Could you check a few things on this model? Use its own coordinates, in mm. A direction names the side the tool comes from. Coordinates: 2 decimals unless noted, no trailing zeros. Order: outer loops, then holes, each group sorted by start corner. A loop starts at its lowest first (then second) coordinate and runs counter-clockwise, first axis right, second up. Notation, with made-up numbers: (53.5, 41.25) - (84.5, 41.25) arc R28 ccw to (84.5, 59.25) - close; hole circle Ø4 at (83, 71). An arc over 180 degrees is marked (long way). One line per item, written item: value. Start each with the question number.
from build123d import *

# Parameters (mm, degrees)
BOSS_EXTRUDE1_DEPTH    = 25.4
CONVERT_SOLID1_DEPTH   = 25.4
CONVERT_SOLID1_2_DEPTH = 25.4
SKETCH7_R              = 2.5019
CUT_EXTRUDE1_DEPTH     = 39.1
FILLET1_R              = 2.54
SKETCH8_R              = 1.89865
CUT_EXTRUDE2_DEPTH     = 38.265357908


# Read off the part's stored shape, not the designer's step: Convert-Solid1
with BuildPart() as part:
    # Sketch2 → Boss-Extrude1 (new body)
    with BuildSketch(Plane.XY):
        Polygon((0, 0), (0, 25.4), (1.27, 25.4), (1.27, 1.27), (12.7, 1.27), (12.7, 0), align=None)
    extrude(amount=BOSS_EXTRUDE1_DEPTH)

    # Convert-Solid1 outline → Convert-Solid1 (cut)
    with BuildSketch(Plane.XY):
        with BuildLine():
            ThreePointArc((2.54, 0), (0.743948776, 0.743948776), (0, 2.54))
            Line((0, 2.54), (0, 0))
            Line((0, 0), (2.54, 0))
        make_face()
    extrude(amount=CONVERT_SOLID1_DEPTH, mode=Mode.SUBTRACT)

    # Convert-Solid1 2 outline → Convert-Solid1 2 (add)
    with BuildSketch(Plane.XY):
        with BuildLine():
            ThreePointArc((2.54, 1.27), (1.641974388, 1.641974388), (1.27, 2.54))
            Line((1.27, 2.54), (1.27, 1.27))
            Line((1.27, 1.27), (2.54, 1.27))
        make_face()
    extrude(amount=CONVERT_SOLID1_2_DEPTH)

    # Sketch7 → Cut-Extrude1 (cut, through all)
    with BuildSketch(Plane.ZY):
        with Locations((12.7, 16.256)):
            Circle(SKETCH7_R)
    extrude(amount=-CUT_EXTRUDE1_DEPTH, mode=Mode.SUBTRACT)

    # Fillet1
    fillet1_edges = [part.edges().sort_by_distance(p)[0] for p in [
        (12.7, 0.635, 0),
        (12.7, 0.635, 25.4),
        (0.635, 25.4, 25.4),
        (0.635, 25.4, 0),
    ]]
    fillet(fillet1_edges, radius=FILLET1_R)

    # Sketch8 → Cut-Extrude2 (cut, through all)
    with BuildSketch(Plane(origin=(0, 1.27, 0), x_dir=(1, 0, 0), z_dir=(0, 1, 0))):
        with Locations(Location((7.62, -5.842, 0), (0, 0, 270))):
            Circle(SKETCH8_R)
        with Locations(Location((7.62, -19.558, 0), (0, 0, 270))):
            Circle(SKETCH8_R)
    extrude(amount=-CUT_EXTRUDE2_DEPTH, mode=Mode.SUBTRACT)


solid = part.part
Q1. We'd pull the mould along Z, two halves only. Please class faces 1 (the flat face through (1, 9, 25.4)), 2 (the cylindrical face through (9.5, 0.64, 5.59)), 3 (the flat face through (0, 11, 13)), 4 (the cylindrical face through (0.63, 17.95, 10.86)): +Z half, -Z half, draft (parallel to the pull), parting line (faces both ways), or undercut.
Q2. I'm going to push flat-ended pins straight in: pin 1 (3 mm diameter, centred on x = 3, z = 11.5, fed in from +Y); pin 2 (6 mm diameter, centred on x = 7, z = 18, fed in from +Y). Where does each tip first touch, or does it pass through?
Q3. I want a section at C-C on z = 22.5. Please give me the cut outline in (x, y).
Q4. I want a section at B-B on x = 7.62. Please give me the cut outline in (y, z).
Q5. I want a section at D-D on y = 15.75. Please give me the cut outline in (x, z).
Q6. Which directions (+Z, -Z, +X, -X, +Y, -Y) give clear straight access to the entire face, cutting with the end or side of a thin tool? Please do faces 5 (the flat face through (1.27, 12, 13)), 6 (the cylindrical face through (0.644, 24.636, 0.724)).
Q7. If I drill on L1, parallel to Y at x = 11.75, z = 11; L2, parallel to X at y = 1.75, z = 12.5, over which ranges is the centre line in solid material (lowest first)?
Q8. I want a section at A-A on z = 12.7. Please give me the cut outline in (x, y), then the cut area to 3 significant figures.
Values follow:
1. face 1: +Z half
1. face 2: undercut
1. face 3: draft
1. face 4: undercut
2. pin 1: stops at y = 1.81
2. pin 2: stops at y = 1.27
3. outline: (0, 2.54) arc R2.54 ccw to (2.54, 0) - (12.7, 0) - (12.7, 1.27) - (2.54, 1.27) arc R1.27 cw to (1.27, 2.54) - (1.27, 25.4) - (0, 25.4) - close
4. outline: (0, 0) - (1.27, 0) - (1.27, 3.94) - (0, 3.94) - close; (0, 7.74) - (1.27, 7.74) - (1.27, 17.66) - (0, 17.66) - close; (0, 21.46) - (1.27, 21.46) - (1.27, 25.4) - (0, 25.4) - close
5. outline: (0, 0) - (1.27, 0) - (1.27, 10.25) - (0, 10.25) - close; (0, 15.15) - (1.27, 15.15) - (1.27, 25.4) - (0, 25.4) - close
6. face 5: +Z, -Z, +X, +Y
6. face 6: -Z, +X, -X, +Y
7. L1: y = 0 to 1.27
7. L2: x = 0.13 to 1.55
8. outline: (0, 2.54) arc R2.54 ccw to (2.54, 0) - (12.7, 0) - (12.7, 1.27) - (2.54, 1.27) arc R1.27 cw to (1.27, 2.54) - (1.27, 13.75) - (0, 13.75) - close; (0, 18.76) - (1.27, 18.76) - (1.27, 25.4) - (0, 25.4) - close
8. area: 39.4 mm^2
